```python
from build123d import *

# Parameters (mm, degrees)
F1_DEPTH      = 5
F1_DEPTH_BACK = 5


with BuildPart() as f1:
    # F0 (on Top) → F1 (new body, two sides)
    with BuildSketch(Plane.XY) as f1_sk:
        Polygon((142.402977, 12), (-154.432267, 12), (-154.432267, -12), (-61.303213, -12), (-50.127726, 2.996326), (-46.240598, 2.996326), (-57.416085, -12), (-36.303213, -12), (-25.127726, 2.996326), (-21.240598, 2.996326), (-32.416085, -12), (-11.303213, -12), (-0.127726, 2.996326), (3.759402, 2.996326), (-7.416085, -12), (13.696787, -12), (24.872274, 2.996326), (28.759402, 2.996326), (17.583915, -12), (38.696787, -12), (49.872274, 2.996326), (53.759402, 2.996326), (42.583915, -12), (142.402977, -12), align=None)
    extrude(amount=F1_DEPTH)
    extrude(f1_sk.sketch, amount=-F1_DEPTH_BACK)


solid = f1.part
```
Geometry check sheet. Reference: the model listing, model coordinates, mm. A direction names the side the tool comes from. Coordinates: 2 decimals unless noted, no trailing zeros. Loops run counter-clockwise (first coordinate to the right, second up) from the corner with the lowest first, then second, coordinate; pieces in that order, holes last.
Item 1: Sectioned sample at A-A, the plane z = 2. Record the boundary of the cut face in (x, y), then the cut area to 3 significant figures.
Item 2: Access from +Z, -Z, +X, -X, +Y, -Y to the whole of each face (thin tool, end or side, straight path). Record for faces 1 (the face through (-5.794, -4.607, 0.07)), 2 (the face through (92, -12, 0)).
Item 3: Release check for a two-part mould opening along X. For faces 3 (the face through (-55.794, -4.607, 0.07)), 4 (the face through (-8, 0, -5)), 5 (the face through (-30.794, -4.607, 0.07)), 6 (the face through (-154.432, 0, 0)) record: released by +X, released by -X, zero draft, split by the parting line, or undercut.
Item 4: Sectioned sample at B-B, the plane y = -8. Record the boundary of the cut face in (x, z).
Item 5: Thickness scan on line 1 (X direction, y = 0, z = -2.5); line 2 (X direction, y = -5, z = 0.75); line 3 (Y direction, x = -26, z = 3). Record the ranges inside material, lowest first.
Check result:
1. outline: (-154.43, -12) - (-61.3, -12) - (-50.13, 3) - (-46.24, 3) - (-57.42, -12) - (-36.3, -12) - (-25.13, 3) - (-21.24, 3) - (-32.42, -12) - (-11.3, -12) - (-0.13, 3) - (3.76, 3) - (-7.42, -12) - (13.7, -12) - (24.87, 3) - (28.76, 3) - (17.58, -12) - (38.7, -12) - (49.87, 3) - (53.76, 3) - (42.58, -12) - (142.4, -12) - (142.4, 12) - (-154.43, 12) - close
1. area: 6,830 mm2
2. face 1: +Z, -Z
2. face 2: +Z, -Z, +X, -X, -Y
3. face 3: undercut
3. face 4: zero draft
3. face 5: undercut
3. face 6: released by -X
4. outline: (-154.43, -5) - (-58.32, -5) - (-58.32, 5) - (-154.43, 5) - close; (-54.44, -5) - (-33.32, -5) - (-33.32, 5) - (-54.44, 5) - close; (-29.44, -5) - (-8.32, -5) - (-8.32, 5) - (-29.44, 5) - close; (-4.44, -5) - (16.68, -5) - (16.68, 5) - (-4.44, 5) - close; (20.56, -5) - (41.68, -5) - (41.68, 5) - (20.56, 5) - close; (45.56, -5) - (142.4, -5) - (142.4, 5) - (45.56, 5) - close
5. line 1: x = -154.43 to -52.36, -48.47 to -27.36, -23.47 to -2.36, 1.53 to 22.64, 26.53 to 47.64, 51.53 to 142.4
5. line 2: x = -154.43 to -56.09, -52.2 to -31.09, -27.2 to -6.09, -2.2 to 18.91, 22.8 to 43.91, 47.8 to 142.4
5. line 3: y = -12 to -3.39, 1.83 to 12
